Geometry: final body of the model. Coordinates: model frame, mm. Face numbers are marked on the shaded views. A direction names the side the tool comes from. Give positions to 0.01 mm unless a question says otherwise; leave off trailing zeros. Write each loop counter-clockwise with the first axis right and the second up, starting at its lowest first coordinate (ties: lowest second). Pieces come first, ordered by that corner, then holes. Notation, with made-up numbers: (-21.75, 80.25) -> (-9.75, 80.25) arc R12 cw to (-9.75, 95.25) -> close; hole circle Ø10 at (40, 40.5). An arc over 180 degrees is marked (long way). Answer in a Markdown table with one row per item. Add a question column.
Item 1: Material intervals for probe 1 along Z at (x, y) = (-10, 12) (3 decimals); probe 2 along Z at (x, y) = (-8.5, 10) (3 decimals); probe 3 along X at (y, z) = (3, -10), sorted ascending. Write a range as from..to.
Item 2: Section query B-B on y = 5. Output: boundary loops of the cut face in (x, z) (3 decimals).
Item 3: First-contact query: P1, Ø3, axis at x = -9.5, z = -11, coming from the +Y side; P2, Ø5, axis at x = -7.71, y = 47.75, coming from the -Z side; P3, Ø2.5, axis at x = 0.5, z = -0.5, coming from the -Y side. Flat tips, straight axial feed; report the tip coordinate or a pass-through.
Item 4: Section query A-A on y = 23.5. Output: boundary loops of the cut face in (x, z) (3 decimals).
Item 5: Section query D-D on x = 5.25. Output: boundary loops of the cut face in (y, z) (1 decimal), plus the area to 3 significant figures.
Item 6: Section query C-C on z = -6.5. Output: boundary loops of the cut face in (x, y).
Item 7: Access query for the marked faces 5, 6 and 7. Directions: +Z, -Z, +X, -X, +Y, -Y. A direction counts if a zero-diameter tool reaches every point of the face in a straight line with its end or side. Return the directions, or none.
Item 8: Draft query along Z for the marked faces 1, 2, 3 and 4. Return one class per face: +Z half, -Z half, draft (parallel to the pull), parting line (faces both ways), or undercut.
```python
from build123d import *

# Parameters (mm, degrees)
SKETCH4_W           = 25.1
SKETCH4_H           = 28.75
BOSS_EXTRUDE2_DEPTH = 53
SKETCH5_W           = 19.1
SKETCH5_H           = 22.75
CUT_EXTRUDE1_DEPTH  = 21.67
FILLET1_R           = 4.1
SKETCH6_W           = 2.88
SKETCH6_H           = 5.1
CUT_EXTRUDE2_DEPTH  = 4.67
SKETCH7_W           = 16.769550268
SKETCH7_H           = 35.14
CUT_EXTRUDE3_DEPTH  = 40
SKETCH8_W           = 13.798322684
SKETCH8_H           = 35.14
CUT_EXTRUDE4_DEPTH  = 40
SKETCH9_W           = 8.5
SKETCH9_H           = 16.46
CUT_EXTRUDE5_DEPTH  = 40
SKETCH10_W          = 10.629287706
SKETCH10_H          = 23.523496481
CUT_EXTRUDE6_DEPTH  = 40
SKETCH11_W          = 25.1
SKETCH11_H          = 2.9448388
CUT_EXTRUDE7_DEPTH  = 16.46
SKETCH14_R          = 1.5
CUT_EXTRUDE10_DEPTH = 23.1
SKETCH13_R          = 1.5
CUT_EXTRUDE11_DEPTH = 23.1


with BuildPart() as part:
    # Sketch4 → Boss-Extrude2 (new body)
    with BuildSketch(Plane(origin=(0, 0, 0), x_dir=(1, 0, 0), z_dir=(0, 1, 0))):
        Rectangle(SKETCH4_W, SKETCH4_H)
    extrude(amount=BOSS_EXTRUDE2_DEPTH)

    # Sketch5 → Cut-Extrude1 (cut)
    with BuildSketch(Plane(origin=(0, 0, 0), x_dir=(-1, 0, 0), z_dir=(0, -1, 0))):
        Rectangle(SKETCH5_W, SKETCH5_H)
    extrude(amount=-CUT_EXTRUDE1_DEPTH, mode=Mode.SUBTRACT)

    # Fillet1
    fillet1_edges = [part.edges().sort_by_distance(p)[0] for p in [
        (0, 21.67, -11.375),
        (0, 21.67, 11.375),
    ]]
    fillet(fillet1_edges, radius=FILLET1_R)

    # Sketch6 → Cut-Extrude2 (cut)
    with BuildSketch(Plane(origin=(0, 21.67, 0), x_dir=(-1, 0, 0), z_dir=(0, -1, 0))):
        Rectangle(SKETCH6_W, SKETCH6_H)
    extrude(amount=-CUT_EXTRUDE2_DEPTH, mode=Mode.SUBTRACT)

    # Sketch7 → Cut-Extrude3 (cut)
    with BuildSketch(Plane(origin=(12.55, 0, 0), x_dir=(0, 0, -1), z_dir=(1, 0, 0))):
        Rectangle(SKETCH7_W, SKETCH7_H)
    extrude(amount=-CUT_EXTRUDE3_DEPTH, mode=Mode.SUBTRACT)

    # Sketch8 → Cut-Extrude4 (cut)
    with BuildSketch(Plane(origin=(0, 0, -14.375), x_dir=(-1, 0, 0), z_dir=(0, 0, -1))):
        Rectangle(SKETCH8_W, SKETCH8_H)
    extrude(amount=-CUT_EXTRUDE4_DEPTH, mode=Mode.SUBTRACT)

    # Sketch9 → Cut-Extrude5 (cut)
    with BuildSketch(Plane.ZY.offset(12.55)):
        with Locations((10.125, 44.77)):
            Rectangle(SKETCH9_W, SKETCH9_H)
    extrude(amount=-CUT_EXTRUDE5_DEPTH, mode=Mode.SUBTRACT)

    # Sketch10 → Cut-Extrude6 (cut)
    with BuildSketch(Plane.ZY.offset(12.55)):
        with Locations((-9.060356147, 41.23825176)):
            Rectangle(SKETCH10_W, SKETCH10_H)
    extrude(amount=-CUT_EXTRUDE6_DEPTH, mode=Mode.SUBTRACT)

    # Sketch11 → Cut-Extrude7 (cut)
    with BuildSketch(Plane(origin=(0, 53, 0), x_dir=(1, 0, 0), z_dir=(0, 1, 0))):
        with Locations((0, -4.4025806)):
            Rectangle(SKETCH11_W, SKETCH11_H)
    extrude(amount=-CUT_EXTRUDE7_DEPTH, mode=Mode.SUBTRACT)

    # Sketch14 → Cut-Extrude10 (cut)
    with BuildSketch(Plane(origin=(0, 0, -3.745712294), x_dir=(-1, 0, 0), z_dir=(0, 0, -1))):
        with Locations((-0.286761368, 47.74761558)):
            Circle(SKETCH14_R)
    extrude(amount=-CUT_EXTRUDE10_DEPTH, mode=Mode.SUBTRACT)

    # Sketch13 → Cut-Extrude11 (cut)
    with BuildSketch(Plane(origin=(0, 0, -3.745712294), x_dir=(-1, 0, 0), z_dir=(0, 0, -1))):
        with Locations((7.713238632, 47.74761558)):
            Circle(SKETCH13_R)
    extrude(amount=-CUT_EXTRUDE11_DEPTH, mode=Mode.SUBTRACT)


solid = part.part
```
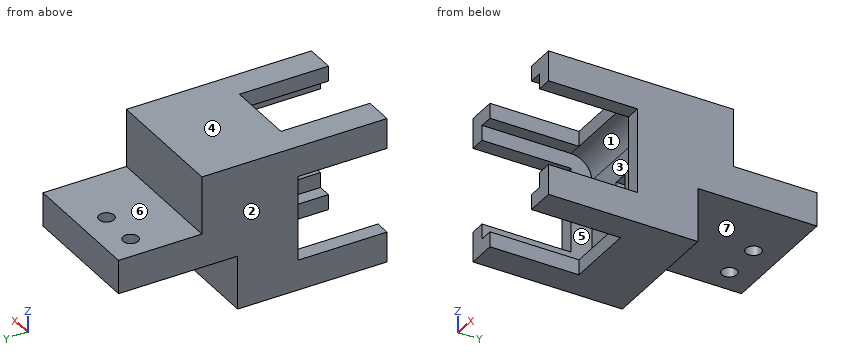
Findings below:
| question | item | result |
|---|---|---|
| 1 | probe 1 | z = -14.375..-8.385, 8.385..14.375 |
| 1 | probe 2 | z = -14.375..-11.375, 11.375..14.375 |
| 1 | probe 3 | x = -12.55..-9.55, 9.55..12.55 |
| 2 | outline | (-12.55, -14.375) -> (-6.899, -14.375) -> (-6.899, -11.375) -> (-9.55, -11.375) -> (-9.55, -8.385) -> (-12.55, -8.385) -> close; (-12.55, 8.385) -> (-9.55, 8.385) -> (-9.55, 11.375) -> (-6.899, 11.375) -> (-6.899, 14.375) -> (-12.55, 14.375) -> close; (6.899, -14.375) -> (12.55, -14.375) -> (12.55, -8.385) -> (9.55, -8.385) -> (9.55, -11.375) -> (6.899, -11.375) -> close; (6.899, 11.375) -> (9.55, 11.375) -> (9.55, 8.385) -> (12.55, 8.385) -> (12.55, 14.375) -> (6.899, 14.375) -> close |
| 3 | P1 | stops at y = 29.48 |
| 3 | P2 | stops at z = -3.75 |
| 3 | P3 | stops at y = 21.67 |
| 4 | outline | (-12.55, -14.375) -> (12.55, -14.375) -> (12.55, 14.375) -> (-12.55, 14.375) -> close; hole (-1.44, -2.55) -> (1.44, -2.55) -> (1.44, 2.55) -> (-1.44, 2.55) -> close |
| 5 | outline | (17.6, -14.4) -> (29.5, -14.4) -> (29.5, -3.7) -> (53, -3.7) -> (53, 2.9) -> (36.5, 2.9) -> (36.5, 14.4) -> (17.6, 14.4) -> (17.6, 11.4) arc R4.1 cw to (21.7, 7.3) -> (21.7, -7.3) arc R4.1 cw to (17.6, -11.4) -> close |
| 5 | area | 494 mm^2 |
| 6 | outline | (-12.55, 17.57) -> (-9.55, 17.57) -> (-9.55, 21.67) -> (9.55, 21.67) -> (9.55, 17.57) -> (12.55, 17.57) -> (12.55, 29.48) -> (-12.55, 29.48) -> close |
| 7 | face 5 | -Y |
| 7 | face 6 | +Z, +X, -X, +Y |
| 7 | face 7 | -Z, +X, -X, +Y |
| 8 | face 1 | undercut |
| 8 | face 2 | draft |
| 8 | face 3 | undercut |
| 8 | face 4 | +Z half |
